For this review, take the finished solid that the model builds, in its own axes (mm). A direction names the side the tool comes from. Round coordinates to 2 decimals unless told otherwise and drop trailing zeros. Loops run counter-clockwise (first coordinate to the right, second up) from the corner with the lowest first, then second, coordinate; pieces in that order, holes last.
1. Consider section C-C on z = 0. State how many separate pieces and enclosed holes the cut face has, then the cut area to 3 significant figures.
2. Consider section B-B on y = 9. State the section outline as (x, z) points.
3. Draft analysis for pull direction Y (two halves, no side actions). For faces 1 (the flat face through (38, 28, 0)), 2 (the flat face through (22, 12, 0)), 3 (the cylindrical face through (2.38, 31.41, 1.83)), state which applies: released by +Y, released by -Y, zero draft, split by the parting line, or undercut.
4. Tool access review of faces 4 (the cylindrical face through (0, 19, 4)), 5 (the flat face through (-22, 13, 0)), 6 (the cylindrical face through (22.5, 29, -0.1)), 7 (the flat face through (38, 19, 0)), 8 (the cylindrical face through (-22.5, 29, -0.1)): name each direction out of +Z, -Z, +X, -X, +Y, -Y from which nothing blocks a thin tool from reaching the whole face with its end or side.
5. Consider section D-D on x = -24.5. State the section outline as (y, z) points, then the cut area to 3 significant figures.
6. Clearance check with flat-ended pins moving along their axes: pin 1 Ø7.5 at (x, z) = (37.5, 0.5) entering from +Y; pin 2 Ø1.5 at (x, z) = (9.5, -7.5) entering from -Y; pin 3 Ø21 at (x, z) = (-33, -4) entering from -Y. State where each tip first meets the part, or that it passes through.
7. Consider section A-A on x = 31. State the section outline as (y, z) points, then the cut area to 3 significant figures.
8. To check wall thickness, follow line 1 along Z through (x, y) = (-31, 24.5); line 2 along Y through (x, z) = (30.5, -15); line 3 along Z through (x, y) = (2, 19). State the ranges of each line that lie inside material, in increasing order.
from build123d import *

# Parameters (mm, degrees)
BOSS_EXTRUDE1_DEPTH                 = 18
F_6_0MM_DOWEL_HOLE1_D               = 9
CUT_EXTRUDE2_DEPTH                  = 10
F_6_0MM_DOWEL_HOLE2_D               = 6
F_6_0MM_DOWEL_HOLE2_DEPTH           = 13
F_6_0MM_DOWEL_HOLE2_TIP             = 3
F_6_0MM_DOWEL_HOLE2_ON_FACE_2_D     = 6
F_6_0MM_DOWEL_HOLE2_ON_FACE_2_DEPTH = 13
F_6_0MM_DOWEL_HOLE2_ON_FACE_2_TIP   = 3
F_5_0MM_DOWEL_HOLE2_D               = 5
CUT_EXTRUDE3_START                  = -23.0000001
CUT_EXTRUDE3_DEPTH                  = 34.000000209


with BuildPart() as part:
    # Sketch1 → Boss-Extrude1 (new body, symmetric)
    with BuildSketch(Plane.XY):
        with BuildLine():
            Line((18.027756377, 6), (22, 6))
            Line((22, 6), (22, 19))
            Line((22, 19), (50, 19))
            Line((50, 19), (50, 28))
            Line((50, 28), (25.690465157, 28))
            ThreePointArc((25.690465157, 28), (0, 38), (-25.690465157, 28))
            Line((-25.690465157, 28), (-50, 28))
            Line((-50, 28), (-50, 19))
            Line((-50, 19), (-22, 19))
            Line((-22, 19), (-22, 6))
            Line((-22, 6), (-18.027756377, 6))
            ThreePointArc((-18.027756377, 6), (0, 19), (18.027756377, 6))
        make_face()
    extrude(amount=BOSS_EXTRUDE1_DEPTH, both=True)

    # Ø6.0mm Dowel Hole1 (through all)
    with Locations(Plane(origin=(0, 28, 0), x_dir=(1, 0, 0), z_dir=(0, 1, 0))):
        with Locations((-31, 0)):
            f_6_0mm_dowel_hole1 = Hole(F_6_0MM_DOWEL_HOLE1_D / 2)

    # Mirror1: Ø6.0mm Dowel Hole1 across plane
    add(f_6_0mm_dowel_hole1.mirror(Plane(origin=(0, 0, 0), x_dir=(0, 0, 1), z_dir=(1, 0, 0))), mode=Mode.SUBTRACT)

    # Sketch6 → Cut-Extrude2 (cut)
    with BuildSketch(Plane(origin=(0, 28, 0), x_dir=(1, 0, 0), z_dir=(0, 1, 0))):
        with BuildLine():
            Line((-25.690465157, -6.637683312), (-25.690465157, 6.637683312))
            ThreePointArc((-25.690465157, 6.637683312), (-22.5, 0), (-25.690465157, -6.637683312))
        make_face()
    cut_extrude2 = extrude(amount=CUT_EXTRUDE2_DEPTH, mode=Mode.SUBTRACT)

    # Mirror3: Cut-Extrude2 across plane
    add(cut_extrude2.mirror(Plane(origin=(0, 0, 0), x_dir=(0, 0, 1), z_dir=(1, 0, 0))), mode=Mode.SUBTRACT)

    # Ø6.0mm Dowel Hole2
    with Locations(Plane(origin=(0.004931503, 37.99999968, 0), x_dir=(0.999999992, -0.000129776, 0), z_dir=(0.000129776, 0.999999992, 0))):
        with Locations((0, 0)):
            Hole(F_6_0MM_DOWEL_HOLE2_D / 2, depth=F_6_0MM_DOWEL_HOLE2_DEPTH)
            with Locations((0, 0, -(F_6_0MM_DOWEL_HOLE2_DEPTH + F_6_0MM_DOWEL_HOLE2_TIP / 2))):  # 90° drill point
                Cone(0, F_6_0MM_DOWEL_HOLE2_D / 2, F_6_0MM_DOWEL_HOLE2_TIP, mode=Mode.SUBTRACT)

    # Ø6.0mm Dowel Hole2 on face 2
    with Locations(Plane(origin=(0, 0, 0), x_dir=(0.999999992, -0.000129776, 0), z_dir=(0.000129776, 0.999999992, 0))):
        with Locations((0, 0)):
            Hole(F_6_0MM_DOWEL_HOLE2_ON_FACE_2_D / 2, depth=F_6_0MM_DOWEL_HOLE2_ON_FACE_2_DEPTH)
            with Locations((0, 0, -(F_6_0MM_DOWEL_HOLE2_ON_FACE_2_DEPTH + F_6_0MM_DOWEL_HOLE2_ON_FACE_2_TIP / 2))):  # 90° drill point
                Cone(0, F_6_0MM_DOWEL_HOLE2_ON_FACE_2_D / 2, F_6_0MM_DOWEL_HOLE2_ON_FACE_2_TIP, mode=Mode.SUBTRACT)

    # Ø5.0mm Dowel Hole2 (through all)
    with Locations(Plane(origin=(-1.0606e-05, 19, 0), x_dir=(-1, -5.58e-07, 0), z_dir=(5.58e-07, -1, 0))):
        with Locations((0, 0)):
            Hole(F_5_0MM_DOWEL_HOLE2_D / 2)

    # Sketch12 → Cut-Extrude3 (cut)
    with BuildSketch(Plane(origin=(0, 28, 0), x_dir=(1, 0, 0), z_dir=(0, 1, 0)).offset(CUT_EXTRUDE3_START)):
        with BuildLine():
            Line((35.09453238, -214.75600598), (-44.497190923, -18))
            ThreePointArc((-44.497190923, -18), (-48, 0), (-44.497190923, 18))
            Line((-44.497190923, 18), (35.09453238, 214.75600598))
            Line((35.09453238, 214.75600598), (-389.394658565, 214.75600598))
            Line((-389.394658565, 214.75600598), (-389.394658565, -214.75600598))
            Line((-389.394658565, -214.75600598), (35.09453238, -214.75600598))
        make_face()
    cut_extrude3 = extrude(amount=CUT_EXTRUDE3_DEPTH, mode=Mode.SUBTRACT)

    # Mirror4: Cut-Extrude3 across plane
    add(cut_extrude3.mirror(Plane(origin=(0, 0, 0), x_dir=(0, 0, 1), z_dir=(1, 0, 0))), mode=Mode.SUBTRACT)


solid = part.part
Resolved:
1. separate pieces: 4
1. enclosed holes: 0
1. area: 1,170 mm2
2. outline: (-22, -18) - (-16.73, -18) - (-16.73, 18) - (-22, 18) - close; (16.73, -18) - (22, -18) - (22, 18) - (16.73, 18) - close
3. face 1: released by +Y
3. face 2: zero draft
3. face 3: undercut
4. face 4: +Z, -Z, -Y
4. face 5: +Z, -Z, -X, -Y
4. face 6: +X, +Y
4. face 7: +Z, -Z, +X, -Y
4. face 8: -X, +Y
5. outline: (19, -18) - (29.05, -18) - (29.05, -5.48) - (28, -5.48) - (28, 5.48) - (29.05, 5.48) - (29.05, 18) - (19, 18) - close
5. area: 350 mm2
6. pin 1: stops at y = 28
6. pin 2: stops at y = 16
6. pin 3: stops at y = 19
7. outline: (19, -18) - (28, -18) - (28, -4.5) - (19, -4.5) - close; (19, 4.5) - (28, 4.5) - (28, 18) - (19, 18) - close
7. area: 243 mm2
8. line 1: z = -18 to -4.5, 4.5 to 18
8. line 2: y = 19 to 28
8. line 3: z = -18 to -1.5, 1.5 to 18
